from build123d import *

# Parameters (mm, degrees)
BOSS_EXTRUDE1_DEPTH = 533
SKETCH2_R           = 22.5
CUT_EXTRUDE1_DEPTH  = 533
SKETCH3_W           = 70
SKETCH3_H           = 59
CUT_EXTRUDE2_DEPTH  = 243


with BuildPart() as part:
    # Sketch1 → Boss-Extrude1 (new body)
    with BuildSketch(Plane.XY):
        Polygon((-344.517995001, 0), (-344.517995001, 499.3), (124.782004999, 499.3), (124.782004999, 0), (124.432004999, 0), (124.432004999, 498.95), (-344.167995001, 498.95), (-344.167995001, 0), align=None)
    extrude(amount=BOSS_EXTRUDE1_DEPTH)

    # Sketch2 → Cut-Extrude1 (cut)
    with BuildSketch(Plane(origin=(124.782004999, 0, 0), x_dir=(0, 0, -1), z_dir=(1, 0, 0))):
        with Locations((-173, 165)):
            Circle(SKETCH2_R)
    extrude(amount=-CUT_EXTRUDE1_DEPTH, mode=Mode.SUBTRACT)

    # Sketch3 → Cut-Extrude2 (cut)
    with BuildSketch(Plane.ZY.offset(344.517995001)):
        with Locations((338, 30.5)):
            Rectangle(SKETCH3_W, SKETCH3_H)
    extrude(amount=-CUT_EXTRUDE2_DEPTH, mode=Mode.SUBTRACT)


solid = part.part
Geometry: final body of the model. Coordinates: model frame, mm. A direction names the side the tool comes from. Coordinates: 2 decimals unless noted, no trailing zeros. Loops run counter-clockwise (first coordinate to the right, second up) from the corner with the lowest first, then second, coordinate; pieces in that order, holes last. Notation, with made-up numbers: (-28.5, 36.25) - (-13.5, 36.25) arc R18 ccw to (-13.5, 57.25) - close; hole circle Ø11 at (68, 84). An arc over 180 degrees is marked (long way). One line per question, with ' | ' between items. Start each with the question number.
(1) Draft query along Z for faces 1 (the flat face through (-113, 499.3, 263)), 2 (the cylindrical face through (-344.34, 171.76, 151.54)). Return one class per face: +Z half, -Z half, draft (parallel to the pull), parting line (faces both ways), or undercut.
(2) Cut plane B-B on z = 173. Output: boundary loops of the cut face in (x, y).
(3) Ray query, L1, parallel to X at y = 65, z = 145.5; L2, parallel to Y at x = 124.65, z = 173; L3, parallel to Y at x = -265, z = 383.5. Return the intervals inside material, ascending. Write a range as from..to.
(4) Cut plane D-D on z = 232.5. Output: boundary loops of the cut face in (x, y), and give its area (3 significant figures).
(5) First-contact query: pin 1 (10 mm diameter, centred on x = -34, z = 395.5, fed in from -Y). Flat tip, straight axial feed; report the tip coordinate or a pass-through.
(6) Cut plane C-C on y = 326. Output: boundary loops of the cut face in (x, z).
(7) Cut plane A-A on y = 165. Output: boundary loops of the cut face in (x, z).
(8) Reachability of faces 3 (the flat face through (-344.168, 253, 263)), 4 (the flat face through (-344.518, 246, 263)) from +Z, -Z, +X, -X, +Y, -Y: full face, straight path, thin tool, end or side. Return the list, or none.
Here are the results:
1) face 1: draft | face 2: undercut
2) outline: (-344.52, 0) - (-344.17, 0) - (-344.17, 142.5) - (-344.52, 142.5) - close; (-344.52, 187.5) - (-344.17, 187.5) - (-344.17, 498.95) - (124.43, 498.95) - (124.43, 187.5) - (124.78, 187.5) - (124.78, 499.3) - (-344.52, 499.3) - close; (124.43, 0) - (124.78, 0) - (124.78, 142.5) - (124.43, 142.5) - close
3) L1: -344.52..-344.17, 124.43..124.78 | L2: 0..142.5, 187.5..499.3 | L3: 498.95..499.3
4) outline: (-344.52, 0) - (-344.17, 0) - (-344.17, 498.95) - (124.43, 498.95) - (124.43, 0) - (124.78, 0) - (124.78, 499.3) - (-344.52, 499.3) - close | area: 514 mm²
5) pin 1: y = 498.95
6) outline: (-344.52, 0) - (-344.17, 0) - (-344.17, 533) - (-344.52, 533) - close; (124.43, 0) - (124.78, 0) - (124.78, 533) - (124.43, 533) - close
7) outline: (-344.52, 0) - (-344.17, 0) - (-344.17, 150.5) - (-344.52, 150.5) - close; (-344.52, 195.5) - (-344.17, 195.5) - (-344.17, 533) - (-344.52, 533) - close; (124.43, 0) - (124.78, 0) - (124.78, 150.5) - (124.43, 150.5) - close; (124.43, 195.5) - (124.78, 195.5) - (124.78, 533) - (124.43, 533) - close
8) face 3: +Z, -Z, -Y | face 4: +Z, -Z, -X, +Y, -Y
